from build123d import *

# Parameters (mm, degrees)
SKETCH1_R           = 38.1
BOSS_EXTRUDE1_DEPTH = 3.175
CUT_EXTRUDE1_DEPTH  = 3.175


with BuildPart() as part:
    # Sketch1 → Boss-Extrude1 (new body)
    with BuildSketch(Plane.XY):
        Circle(SKETCH1_R)
    extrude(amount=BOSS_EXTRUDE1_DEPTH)

    # Sketch2 → Cut-Extrude1 (cut)
    with BuildSketch(Plane.XY):
        Polygon((0, 17.78), (12.7, 17.78), (12.7, 20.955), (-12.7, 20.955), (-12.7, 17.78), align=None)
        Polygon((0, -17.78), (12.7, -17.78), (12.7, -20.955), (-12.7, -20.955), (-12.7, -17.78), align=None)
        Polygon((-28.575, 0), (-28.575, -6.35), (-31.75, -6.35), (-31.75, 6.35), (-28.575, 6.35), align=None)
        Polygon((28.575, 0), (28.575, 6.35), (31.75, 6.35), (31.75, -6.35), (28.575, -6.35), align=None)
    extrude(amount=CUT_EXTRUDE1_DEPTH, mode=Mode.SUBTRACT)


solid = part.part
Could you check a few things on this model? Use its own coordinates, in mm. A direction names the side the tool comes from. Round coordinates to 2 decimals unless told otherwise and drop trailing zeros. Order: outer loops, then holes, each group sorted by start corner. A loop starts at its lowest first (then second) coordinate and runs counter-clockwise, first axis right, second up.
(1) I'm going to push flat-ended pins straight in: pin 1 (1 mm diameter, centred on y = 19.5, z = 1, fed in from -X); pin 2 (1.6 mm diameter, centred on x = -30, z = 2.5, fed in from -Y); pin 3 (1.6 mm diameter, centred on y = 2.5, z = 1, fed in from +X). Where does each tip first touch, or does it pass through?
Response values:
pin 1: stops at x = -33.02
pin 2: stops at y = -24.47
pin 3: stops at x = 38.06
(2) If we mould it in two halves opening along Y, with no side actions, what happens to faces 1 (the cylindrical face through (-30.235, -23.183, 1.565)), 2 (the flat face through (-31.75, 0, 2)), 3 (the flat face through (0, -20.955, 2)), 4 (the flat face through (-1, 1, 0))? For each: released by +Y, released by -Y, zero draft, split by the parting line, or undercut.
Response values:
face 1: split by the parting line
face 2: undercut
face 3: undercut
face 4: zero draft
(3) Imagine slicing it at A-A (y = 0). Write out the boundary of the cut face in (x, z) (3 decimals), plus the area to 3 significant figures.
Response values:
outline: (-38.1, 0) - (-31.75, 0) - (-31.75, 3.175) - (-38.1, 3.175) - close; (-28.575, 0) - (28.575, 0) - (28.575, 3.175) - (-28.575, 3.175) - close; (31.75, 0) - (38.1, 0) - (38.1, 3.175) - (31.75, 3.175) - close
area: 222 mm2
(4) Imagine slicing it at D-D (y = 8). Write out the boundary of the cut face in (x, z) (3 decimals).
Response values:
outline: (-37.251, 0) - (37.251, 0) - (37.251, 3.175) - (-37.251, 3.175) - close
(5) Imagine slicing it at B-B (z = 0.5). Write out the boundary of the cut face in (x, y) (3 decimals).
Response values:
outline: circle Ø76.2 at (0, 0); hole (-31.75, -6.35) - (-28.575, -6.35) - (-28.575, 6.35) - (-31.75, 6.35) - close; hole (-12.7, -20.955) - (12.7, -20.955) - (12.7, -17.78) - (-12.7, -17.78) - close; hole (-12.7, 17.78) - (12.7, 17.78) - (12.7, 20.955) - (-12.7, 20.955) - close; hole (28.575, -6.35) - (31.75, -6.35) - (31.75, 6.35) - (28.575, 6.35) - close
(6) Which directions (+Z, -Z, +X, -X, +Y, -Y) give clear straight access to the entire face, cutting with the end or side of a thin tool? Please do faces 5 (the flat face through (30, 6.35, 2)), 6 (the flat face through (-1, 1, 3.175)).
Response values:
face 5: +Z, -Z
face 6: +Z, +X, -X, +Y, -Y
(7) Please list where these lines run through material, in increasing order: line 1 along Y through (x, z) = (0, 2.2) (3 decimals); line 2 along Y through (x, z) = (-3, 1.55) (3 decimals); line 3 along Y through (x, z) = (-29, 2.5).
Response values:
line 1: y = -38.1 to -20.955, -17.78 to 17.78, 20.955 to 38.1
line 2: y = -37.982 to -20.955, -17.78 to 17.78, 20.955 to 37.982
line 3: y = -24.71 to -6.35, 6.35 to 24.71
(8) Imagine slicing it at C-C (x = 0). Write out the boundary of the cut face in (y, z) (3 decimals), plus the area to 3 significant figures.
Response values:
outline: (-38.1, 0) - (-20.955, 0) - (-20.955, 3.175) - (-38.1, 3.175) - close; (-17.78, 0) - (17.78, 0) - (17.78, 3.175) - (-17.78, 3.175) - close; (20.955, 0) - (38.1, 0) - (38.1, 3.175) - (20.955, 3.175) - close
area: 222 mm2
